Read the model definition and answer for the solid it produces. Units are mm, in the model's axes. A direction names the side the tool comes from. Coordinates: 2 decimals unless noted, no trailing zeros. Loops run counter-clockwise (first coordinate to the right, second up) from the corner with the lowest first, then second, coordinate; pieces in that order, holes last.
from build123d import *

# Parameters (mm, degrees)
F0_W     = 193
F0_H     = 40.3
F1_DEPTH = 2
F3_DEPTH = 1


with BuildPart() as f1:
    # F0 (on Top) → F1 (new body)
    with BuildSketch(Plane.XY):
        with Locations((1.831396, -32.759346)):
            Rectangle(F0_W, F0_H)
    extrude(amount=F1_DEPTH)

    # F2 (on face) → F3 (cut)
    with BuildSketch(Plane.XY.offset(2)):
        Polygon((-53.375542, -25.216417), (-84.645547, -16.741371), (-32.626286, -44.212215), (-32.626286, -35.444923), (7.411011, -46.550158), (7.411011, -35.444923), (47.740549, -47.719132), (47.740549, -35.444923), (91.284759, -45.67343), (33.420641, -14.987911), (33.420641, -25.216417), (-12.169273, -13.818938), (-12.169273, -25.216417), (-53.375542, -14.695669), align=None)
    extrude(amount=-F3_DEPTH, mode=Mode.SUBTRACT)


solid = f1.part
Item 1: Find the intervals of material crossed by line 1 along Y through (x, z) = (53.5, 1.25); line 2 along Y through (x, z) = (-48.5, 1.4); line 3 along X through (y, z) = (-33, 1.9), in increasing order.
Numbers:
line 1: y = -52.91 to -36.8, -25.64 to -12.61
line 2: y = -52.91 to -35.83, -15.94 to -12.61
line 3: x = -94.67 to -53.86, 67.39 to 98.33
Item 2: Determine the mould class of faces 1 (the face through (-12.89, -40.92, 1.51)), 2 (the face through (0, -46, 2)) for opening direction Y: released by +Y, released by -Y, zero draft, split by the parting line, or undercut.
Numbers:
face 1: undercut
face 2: zero draft
Item 3: A cutting plane is placed at A-A on z = 1.3. Determine the outline of the cut face in (x, y).
Numbers:
outline: (-94.67, -52.91) - (98.33, -52.91) - (98.33, -12.61) - (-94.67, -12.61) - close; hole (-84.65, -16.74) - (-32.63, -44.21) - (-32.63, -35.44) - (7.41, -46.55) - (7.41, -35.44) - (47.74, -47.72) - (47.74, -35.44) - (91.28, -45.67) - (33.42, -14.99) - (33.42, -25.22) - (-12.17, -13.82) - (-12.17, -25.22) - (-53.38, -14.7) - (-53.38, -25.22) - close
Item 4: Which of the six approach directions +Z, -Z, +X, -X, +Y, -Y give full straight-line access (tool end or side, diameter ignored) to faces 3 (the face through (0, -32, 0)), 4 (the face through (10.945, -19.597, 1.507))?
Numbers:
face 3: -Z, +X, -X, +Y, -Y
face 4: +Z
Item 5: A cutting plane is placed at D-D on y = -23. Determine the outline of the cut face in (x, z).
Numbers:
outline: (-94.67, 0) - (98.33, 0) - (98.33, 2) - (48.53, 2) - (48.53, 1) - (33.42, 1) - (33.42, 2) - (24.55, 2) - (24.55, 1) - (-12.17, 1) - (-12.17, 2) - (-20.85, 2) - (-20.85, 1) - (-53.38, 1) - (-53.38, 2) - (-61.55, 2) - (-61.55, 1) - (-72.79, 1) - (-72.79, 2) - (-94.67, 2) - close
Item 6: Given pin 1 (1 mm diameter, centred on x = -24.5, y = -29.5, fed in from +Z), flat-ended and moving along its own axis, determine where the tip first touches the part or whether it passes through.
Numbers:
pin 1: stops at z = 1
Item 7: A cutting plane is placed at B-B on y = -42.5. Determine the outline of the cut face in (x, z), then the cut area to 3 significant figures.
Numbers:
outline: (-94.67, 0) - (98.33, 0) - (98.33, 2) - (85.3, 2) - (85.3, 1) - (77.78, 1) - (77.78, 2) - (47.74, 2) - (47.74, 1) - (30.59, 1) - (30.59, 2) - (7.41, 2) - (7.41, 1) - (-7.19, 1) - (-7.19, 2) - (-32.63, 2) - (-32.63, 1) - (-35.87, 1) - (-35.87, 2) - (-94.67, 2) - close
area: 343 mm2
Item 8: A cutting plane is placed at C-C on x = -74. Determine the outline of the cut face in (y, z), then the cut area to 3 significant figures.
Numbers:
outline: (-52.91, 0) - (-12.61, 0) - (-12.61, 2) - (-19.63, 2) - (-19.63, 1) - (-22.36, 1) - (-22.36, 2) - (-52.91, 2) - close
area: 77.9 mm2
